Build history of the part. All positions in model axes, mm. Face numbers are marked on the shaded views. Give positions to 0.01 mm unless a question says otherwise; leave off trailing zeros. Loops run counter-clockwise (first coordinate to the right, second up) from the corner with the lowest first, then second, coordinate; pieces in that order, holes last. Notation, with made-up numbers: (-6.75, 26) -> (6.25, 26) arc R22 cw to (6.25, 63) -> close; hole circle Ø5 at (29, 32). An arc over 180 degrees is marked (long way). Answer as a JSON object with one key per item and string values. Group by question number.
Q1. Wall check: probe 1 along Y at (x, z) = (-8.25, 0); probe 2 along X at (y, z) = (11.5, 1.5); probe 3 along Y at (x, z) = (2.25, 0). Give the ranges that are in metal, low to high. Write a range as from..to.
Q2. Band-saw the part on B-B, the plane x = 6.5. Write the cut outline in (y, z).
Q3. Drop flat-ended pins along their axis: pin 1 (12 mm diameter, centred on x = -1.5, y = -2, fed in from -Z); pin 2 (4 mm diameter, centred on x = 2, y = -9.5, fed in from -Z); pin 3 (8 mm diameter, centred on x = 5, z = -9, fed in from +Y); pin 4 (1 mm diameter, centred on y = 0, z = 0.5, fed in from +X). Give the stop position or say it passes through.
Q4. Two-plate mould, pull along Y, no slides. Class the marked faces 1, 2, 3 and 4: pulls with the +Y half, pulls with the -Y half, needs draft (parallel to the pull), parting line crosses it, or undercut.
Q5. Band-saw the part on C-C, the plane x = -6.5. Write the cut outline in (y, z), plus the area to 3 significant figures.
Q6. Band-saw the part on A-A, the plane z = 0. Count the separate pieces of the cut face and the enclosed holes in it, plus the area to 3 significant figures.
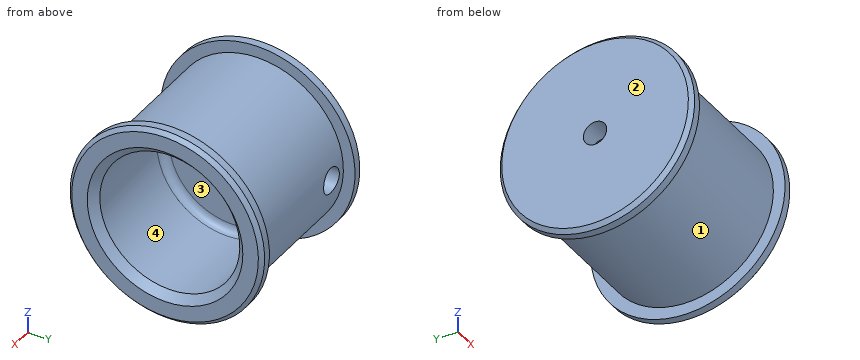
from build123d import *

# Parameters (mm, degrees)
REBAIXO_PARA_PARAFUSO_DE_M_QUINA_DE_CABE_D           = 3
REBAIXO_PARA_PARAFUSO_DE_M_QUINA_DE_CABE_CBORE_D     = 18
REBAIXO_PARA_PARAFUSO_DE_M_QUINA_DE_CABE_CBORE_DEPTH = 14
FURO_DE_DI_METRO_3_3_3_3_1_OUTLINE_R                 = 1.65
FURO_DE_DI_METRO_3_3_3_3_1_DEPTH                     = 11.000000058
CHANFRO1_SIZE                                        = 0.5
CHANFRO2_SIZE                                        = 1
FILETE1_R                                            = 1


# Read off the part's stored shape, not the designer's step: Furo de diâmetro Ø3.3 (3.3)1
with BuildPart() as part:
    # Esboço1 → Revolução1 (revolve)
    with BuildSketch(Plane(origin=(0, 0, 0), x_dir=(-1, 0, 0), z_dir=(0, 0, -1)), mode=Mode.PRIVATE) as revolu_o1_sk:
        Polygon((-10.5, 12.5), (-10.5, 0), (10.5, 0), (10.5, 12.5), (9, 12.5), (9, 11), (-9, 11), (-9, 12.5), align=None)
    revolve(revolu_o1_sk.sketch.rotate(Axis((10.5, 0, 0), (-1, 0, 0)), 270), axis=Axis((10.5, 0, 0), (-1, 0, 0)))

    # Rebaixo para parafuso de máquina de cabeça sextavada de M2.51 (through all)
    with Locations(Plane(origin=(10.5, 0, 0), x_dir=(0, 0, -1), z_dir=(1, 0, 0))):
        with Locations((0, 0)):
            CounterBoreHole(REBAIXO_PARA_PARAFUSO_DE_M_QUINA_DE_CABE_D / 2, REBAIXO_PARA_PARAFUSO_DE_M_QUINA_DE_CABE_CBORE_D / 2, REBAIXO_PARA_PARAFUSO_DE_M_QUINA_DE_CABE_CBORE_DEPTH)

    # Furo de diâmetro Ø3.3 (3.3)1 outline → Furo de diâmetro Ø3.3 (3.3)1 (cut)
    with BuildSketch(Plane(origin=(0, 0, 0), x_dir=(1, 0, 0), z_dir=(0, 1, 0))):
        with Locations((-6.5, 0)):
            Circle(FURO_DE_DI_METRO_3_3_3_3_1_OUTLINE_R)
    extrude(amount=FURO_DE_DI_METRO_3_3_3_3_1_DEPTH, mode=Mode.SUBTRACT)

    # Chanfro1
    chanfro1_edges = [part.edges().sort_by_distance(p)[0] for p in [
        (10.5, 0, -12.5),
        (-10.5, 0, -12.5),
    ]]
    chamfer(chanfro1_edges, length=CHANFRO1_SIZE)

    # Chanfro2
    chanfro2_edges = [part.edges().sort_by_distance(p)[0] for p in [
        (10.5, 0, 9),
    ]]
    chamfer(chanfro2_edges, length=CHANFRO2_SIZE)

    # Filete1
    filete1_edges = [part.edges().sort_by_distance(p)[0] for p in [
        (-3.5, 0, 9),
    ]]
    fillet(filete1_edges, radius=FILETE1_R)


solid = part.part
Worked answers:
{
 "1": {"probe 1": "-11..-1.5, 1.5..11", "probe 2": "-10.5..-9, 9..10.5", "probe 3": "-11..-9, 9..11"},
 "2": {"outline": "circle Ø22 at (0, 0); hole circle Ø18 at (0, 0)"},
 "3": {"pin 1": "z = -11", "pin 2": "z = -8.05", "pin 3": "y = 9.8", "pin 4": "through"},
 "4": {"face 1": "parting line crosses it", "face 2": "needs draft", "face 3": "undercut", "face 4": "undercut"},
 "5": {"outline": "(0, -1.65) -> (0, -1.5) arc R1.5 cw to (0, 1.5) -> (0, 1.65) -> (10.88, 1.65) arc R11 ccw (long way) to (10.88, -1.65) -> close", "area": "340 mm2"},
 "6": {"separate pieces": "3", "enclosed holes": "0", "area": "166 mm2"}
}
